Read the model definition and answer for the solid it produces. Units are mm, in the model's axes. Face numbers are marked on the shaded views. A direction names the side the tool comes from. Give positions to 0.01 mm unless a question says otherwise; leave off trailing zeros. Loops run counter-clockwise (first coordinate to the right, second up) from the corner with the lowest first, then second, coordinate; pieces in that order, holes last. Notation, with made-up numbers: (60, 38.25) -> (100, 38.25) arc R20 cw to (100, 67.25) -> close; hole circle Ø2 at (60.5, -34.5). An arc over 180 degrees is marked (long way). Write each question's results on one line, items separated by ' | '. Start each with the question number.
Item 1: Which of the six approach directions +Z, -Z, +X, -X, +Y, -Y give full straight-line access (tool end or side, diameter ignored) to the marked faces 1 and 2?
Item 2: Section A-A on z = 0 is taken. Write down the section's boundary in (x, y).
Item 3: Each of these flat-tipped pins is pushed along its axis until it touches: P1, Ø6, axis at x = 1.5, y = 4.5, coming from the +Z side; P2, Ø5, axis at y = -2, z = -1.5, coming from the +X side; P3, Ø3, axis at x = 11, y = 1.5, coming from the +Z side; P4, Ø5, axis at x = 4.5, y = 3.5, coming from the -Z side. Where does it stop, or does it pass through?
Item 4: Find the intervals of material crossed by line 1 (X direction, y = -3, z = 2.5); line 2 (Z direction, x = 5, y = 1); line 3 (Z direction, x = 2.25, y = 5.75), in increasing order.
Item 5: Section C-C on x = 6 is taken. Write down the section's boundary in (y, z), and give its area (3 significant figures).
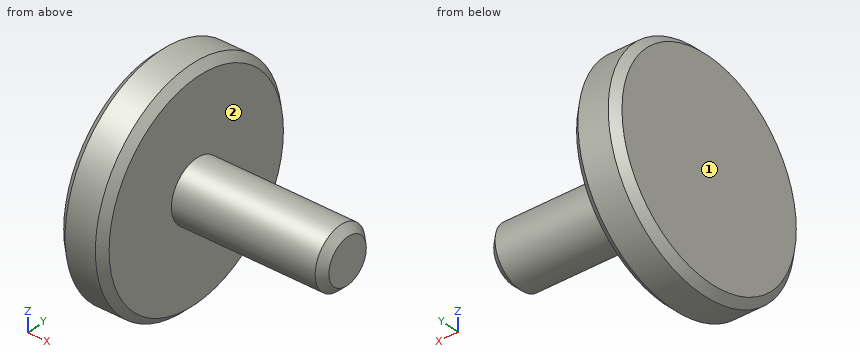
```python
from build123d import *

# Parameters (mm, degrees)
CHANFREIN1_SIZE = 0.5


with BuildPart() as part:
    # Esquisse1 → Révolution1 (revolve)
    with BuildSketch(Plane.XY, mode=Mode.PRIVATE) as r_volution1_sk:
        Polygon((0, 0), (0, 7.5), (3, 7.5), (3, 2), (13, 2), (13, 0), align=None)
    revolve(r_volution1_sk.sketch.rotate(Axis((-65.170410524, 0, 0), (1, 0, 0)), 90), axis=Axis((-65.170410524, 0, 0), (1, 0, 0)))

    # Chanfrein1
    chanfrein1_edges = [part.edges().sort_by_distance(p)[0] for p in [
        (13, 0, -2),
        (3, 0, -7.5),
        (0, 0, -7.5),
    ]]
    chamfer(chanfrein1_edges, length=CHANFREIN1_SIZE)


solid = part.part
```
Findings:
1) face 1: +Z, -Z, -X, +Y, -Y | face 2: +X
2) outline: (0, -7) -> (0.5, -7.5) -> (2.5, -7.5) -> (3, -7) -> (3, -2) -> (12.5, -2) -> (13, -1.5) -> (13, 1.5) -> (12.5, 2) -> (3, 2) -> (3, 7) -> (2.5, 7.5) -> (0.5, 7.5) -> (0, 7) -> close
3) P1: z = 7.35 | P2: x = 13 | P3: z = 2 | P4: z = -7.23
4) line 1: 0 to 3 | line 2: -1.73 to 1.73 | line 3: -4.82 to 4.82
5) outline: circle Ø4 at (0, 0) | area: 12.6 mm2
